```python
from build123d import *

# Parameters (mm, degrees)
F3_DEPTH     = 31.75
F5_DEPTH     = 6.35
F6_SIZE      = 12.7
F7_SIZE      = 12.7
F9_DEPTH     = 31.75
F11_DEPTH    = 12.7
F13_T2_ANGLE = 48.1784563201
F13_T4_ANGLE = 86.2150976381
F13_T6_ANGLE = 86.2150976381
F13_T8_ANGLE = 48.1784563201
F15_DEPTH    = 12.7
F16_SIZE     = 5.08
F18_DEPTH    = 2.54
F20_DEPTH    = 2.54
F21_R        = 7.62
F22_DEPTH    = 38.1
F24_DEPTH    = 2.794
F26_DEPTH    = 2.54
F27_R        = 10.16
F27_R_2      = 9.525
F28_DEPTH    = 76.2


# Not quite as in the source:
# - a fillet or chamfer that OpenCascade refuses, or shapes differently, is made with other operations: its cross-section is extruded or revolved along the edge and cut away or added
# - a feature of the source that left no trace in its solid (it failed there, or was rolled back) is left out
# - a feature names something its author has since deleted; it is built from what else it names


with BuildPart() as f3:
    # F2 (on Front) → F3 (new body, symmetric)
    with BuildSketch(Plane.XZ):
        with BuildLine():
            Line((37.9477068782, 57.15), (37.9477068782, -69.85))
            ThreePointArc((37.9477068782, -69.85), (197.3095607255, -116.6415507663), (342.7477068782, -196.85))
            Line((342.7477068782, -196.85), (342.7477068782, -156.4439684153))
            Line((342.7477068782, -156.4439684153), (333.764821291, -146.2200134993))
            Line((333.764821291, -146.2200134993), (333.764821291, -76.4565169811))
            Line((333.764821291, -76.4565169811), (299.7545793033, -41.7148783095))
            ThreePointArc((299.7545793033, -41.7148783095), (173.42869903, 19.8395158234), (37.9477068782, 57.15))
        make_face()
    extrude(amount=F3_DEPTH, both=True)

    # F4 (on Front) → F5 (cut, symmetric)
    with BuildSketch(Plane.XZ):
        with BuildLine():
            Line((37.9477068782, -48.4879799187), (37.9477068782, -69.85))
            ThreePointArc((37.9477068782, -69.85), (197.3095607255, -116.6415507663), (342.7477068782, -196.85))
            Line((342.7477068782, -196.85), (342.7477068782, -156.4439684153))
            Line((342.7477068782, -156.4439684153), (333.764821291, -146.2200134993))
            Line((333.764821291, -146.2200134993), (333.764821291, -76.4565169811))
            Line((333.764821291, -76.4565169811), (299.7545793033, -41.7148783095))
            ThreePointArc((299.7545793033, -41.7148783095), (173.42869903, 19.8395158234), (37.9477068782, 57.15))
            Line((37.9477068782, 57.15), (37.9477068782, 40.4159426689))
            ThreePointArc((37.9477068782, 40.4159426689), (174.1077804995, -9.1728518585), (291.3761138916, -94.3007096648))
            Line((291.3761138916, -94.3007096648), (297.9114055634, -145.1900005341))
            ThreePointArc((297.9114055634, -145.1900005341), (173.776538026, -81.1205697987), (37.9477068782, -48.4879799187))
        make_face()
    extrude(amount=F5_DEPTH, both=True, mode=Mode.SUBTRACT)

    # F6
    f6_edges = [f3.edges().sort_by_distance(p)[0] for p in [
        (173.428699, -31.75, 19.839516),
        (316.7597, -31.75, -59.085698),
        (316.7597, 31.75, -59.085698),
        (173.428699, 31.75, 19.839516),
    ]]
    chamfer(f6_edges, length=F6_SIZE)

    # F7
    f7_edges = [f3.edges().sort_by_distance(p)[0] for p in [
        (197.309561, -31.75, -116.641551),
        (197.309561, 31.75, -116.641551),
    ]]
    chamfer(f7_edges, length=F7_SIZE)

    # F8 (on Front) → F9 (join, symmetric)
    with BuildSketch(Plane.XZ):
        with BuildLine():
            ThreePointArc((86.9189181185, -80.2493599938), (62.5187399917, -74.647396796), (37.9477068782, -69.85))
            Line((37.9477068782, -69.85), (37.9477068782, -171.45))
            ThreePointArc((37.9477068782, -171.45), (117.3693749826, -201.1045334968), (188.127681613, -247.7998733521))
            ThreePointArc((188.127681613, -247.7998733521), (259.6802456544, -259.033648506), (329.51571574, -278.2423507795))
            Line((329.51571574, -278.2423507795), (342.7477068782, -203.2))
            ThreePointArc((342.7477068782, -203.2), (210.1366349445, -151.4972629597), (86.9189181185, -80.2493599938))
        make_face()
        with BuildLine():
            add(Edge.make_bspline(
                [(37.9477068782, -69.85), (37.9477068782, -67.7549506267), (37.9477068782, -65.6599012534), (37.9477068782, -63.5648518801)],
                knots=[0, 0, 0, 0, 0.4873412151, 0.4873412151, 0.4873412151, 0.4873412151], degree=3))
            ThreePointArc((37.9477068782, -69.85), (62.5187399917, -74.647396796), (86.9189181185, -80.2493599938))
            ThreePointArc((86.9189181185, -80.2493599938), (75.0688400161, -71.9981901024), (63.3477068782, -63.5648518801))
            Line((63.3477068782, -63.5648518801), (37.9477068782, -63.5648518801))
        make_face()
    extrude(amount=F9_DEPTH, both=True)

    # F10 (on Front) → F11 (cut, symmetric)
    with BuildSketch(Plane.XZ):
        with BuildLine():
            add(Edge.make_bspline(
                [(37.9477068782, -69.85), (37.9477068782, -67.7549506267), (37.9477068782, -65.6599012534), (37.9477068782, -63.5648518801)],
                knots=[0, 0, 0, 0, 0.4873412151, 0.4873412151, 0.4873412151, 0.4873412151], degree=3))
            Line((37.9477068782, -69.85), (37.9477068782, -171.45))
            ThreePointArc((37.9477068782, -171.45), (117.3693749826, -201.1045334968), (188.127681613, -247.7998733521))
            ThreePointArc((188.127681613, -247.7998733521), (259.6802456544, -259.033648506), (329.51571574, -278.2423507795))
            Line((329.51571574, -278.2423507795), (342.7477068782, -203.2))
            ThreePointArc((342.7477068782, -203.2), (197.1706361591, -145.1420264492), (63.3477068782, -63.5648518801))
            Line((63.3477068782, -63.5648518801), (37.9477068782, -63.5648518801))
        make_face()
    extrude(amount=F11_DEPTH, both=True, mode=Mode.SUBTRACT)

    # F13: chamfer of 76.2 x 19.05 on 4 edges, made by hand

    # F13_s1 → F13_t2 (revolve, cut)
    with BuildSketch(Plane(origin=(-60.6535291513, 0, -12.8240400006), x_dir=(0, 1, 0), z_dir=(-0.9783709739, 0, -0.2068580127))):
        Polygon((31.75, 174.9435450059), (12.7, 251.1435450059), (31.75, 251.1435450059), align=None)
    revolve(axis=Axis((124.3217755456, 31.75, -887.6969377111), (0, 1, 0)), revolution_arc=F13_T2_ANGLE, mode=Mode.SUBTRACT)

    # F13_s3 → F13_t4 (revolve, cut)
    with BuildSketch(Plane(origin=(-192.2531449662, 0, -55.7064857223), x_dir=(0, 1, 0), z_dir=(-0.9604918286, 0, -0.2783081876))):
        Polygon((12.7, 124.3402407106), (31.75, 48.1402407106), (31.75, 124.3402407106), align=None)
    revolve(axis=Axis((-53.0135938756, 31.75, -536.2473285656), (0, 1, 0)), revolution_arc=F13_T4_ANGLE, mode=Mode.SUBTRACT)

    # F13_s5 → F13_t6 (revolve, cut)
    with BuildSketch(Plane(origin=(-192.2531449662, 0, -55.7064857223), x_dir=(0, 1, 0), z_dir=(-0.9604918286, 0, -0.2783081876))):
        Polygon((-31.75, 48.1402407106), (-12.7, 124.3402407106), (-31.75, 124.3402407106), align=None)
    revolve(axis=Axis((-53.0135938756, -31.75, -536.2473285656), (0, 1, 0)), revolution_arc=F13_T6_ANGLE, mode=Mode.SUBTRACT)

    # F13_s7 → F13_t8 (revolve, cut)
    with BuildSketch(Plane(origin=(-60.6535291513, 0, -12.8240400006), x_dir=(0, 1, 0), z_dir=(-0.9783709739, 0, -0.2068580127))):
        Polygon((-31.75, 174.9435450059), (-12.7, 251.1435450059), (-31.75, 251.1435450059), align=None)
    revolve(axis=Axis((124.3217755456, -31.75, -887.6969377111), (0, 1, 0)), revolution_arc=F13_T8_ANGLE, mode=Mode.SUBTRACT)

    # F14 (on Front) → F15 (join, symmetric)
    with BuildSketch(Plane.XZ):
        with BuildLine():
            Line((354.91571574, -208.3923507795), (354.91571574, -113.1423507795))
            ThreePointArc((354.91571574, -113.1423507795), (259.66571574, -208.3923507795), (354.91571574, -303.6423507795))
            Line((354.91571574, -303.6423507795), (354.91571574, -208.3923507795))
        make_face()
    extrude(amount=F15_DEPTH, both=True)

    # F16
    f16_edges = [f3.edges().sort_by_distance(p)[0] for p in [
        (310.909323, -12.7, -292.867199),
        (270.087911, -12.7, -165.070232),
        (344.273637, -12.7, -113.738726),
        (344.273637, 12.7, -113.738726),
        (270.087911, 12.7, -165.070232),
        (310.909323, 12.7, -292.867199),
    ]]
    chamfer(f16_edges, length=F16_SIZE)

    # F17 (on face) → F18 (cut)
    with BuildSketch(Plane.XZ.offset(31.75)):
        with BuildLine():
            Line((37.9477068782, 18.4170784308), (37.9477068782, -18.7770907031))
            Line((37.9477068782, -18.7770907031), (44.5238578239, -19.4250085564))
            ThreePointArc((44.5238578239, -19.4250085564), (166.0160786587, -50.5371993601), (281.275870441, -99.9690568843))
            Line((281.275870441, -99.9690568843), (270.4956403873, -68.620350335))
            ThreePointArc((270.4956403873, -68.620350335), (157.9813255542, -15.0565404403), (37.9477068782, 18.4170784308))
        make_face()
    extrude(amount=-F18_DEPTH, mode=Mode.SUBTRACT)

    # F19 (on face) → F20 (cut)
    with BuildSketch(Plane(origin=(0, 31.75, 0), x_dir=(-1, 0, 0), z_dir=(0, 1, 0))):
        with BuildLine():
            ThreePointArc((-37.9477068782, 18.4170784308), (-157.9813255542, -15.0565404403), (-270.4956403873, -68.620350335))
            Line((-270.4956403873, -68.620350335), (-281.275870441, -99.9690568843))
            ThreePointArc((-281.275870441, -99.9690568843), (-166.0160786587, -50.5371993601), (-44.5238578239, -19.4250085564))
            Line((-44.5238578239, -19.4250085564), (-37.9477068782, -18.7770907031))
            Line((-37.9477068782, -18.7770907031), (-37.9477068782, 18.4170784308))
        make_face()
    extrude(amount=-F20_DEPTH, mode=Mode.SUBTRACT)

    # F21 (on face) → F22 (cut)
    with BuildSketch(Plane.YZ.offset(354.91571574)):
        with Locations((0, -208.3923507795)):
            Circle(F21_R)
    extrude(amount=-F22_DEPTH, mode=Mode.SUBTRACT)

    # F23 (on face) → F24 (cut)
    with BuildSketch(Plane.XZ.offset(12.7)):
        with BuildLine():
            ThreePointArc((331.4293971954, -267.3893239326), (342.9586633277, -270.7564341738), (354.91571574, -271.8923507795))
            Line((354.91571574, -271.8923507795), (354.91571574, -259.1923507795))
            ThreePointArc((354.91571574, -259.1923507795), (344.0535486893, -258.0174787588), (333.6938090461, -254.5472061718))
            Line((333.6938090461, -254.5472061718), (331.4293971954, -267.3893239326))
        make_face()
        with BuildLine():
            ThreePointArc((342.7477068782, -159.0711630369), (348.7869449547, -157.9634090034), (354.91571574, -157.5923507795))
            Line((354.91571574, -157.5923507795), (354.91571574, -144.8923507795))
            ThreePointArc((354.91571574, -144.8923507795), (344.9966028413, -145.6718501493), (335.3210156829, -147.991210644))
            Line((335.3210156829, -147.991210644), (342.7477068782, -156.4439684153))
            Line((342.7477068782, -156.4439684153), (342.7477068782, -159.0711630369))
        make_face()
        with BuildLine():
            ThreePointArc((303.5618689691, -171.0422179573), (298.710555552, -178.8418860075), (295.0352686554, -187.2598625929))
            ThreePointArc((295.0352686554, -187.2598625929), (301.0091143651, -189.413157651), (306.9974582895, -191.5257979926))
            ThreePointArc((306.9974582895, -191.5257979926), (310.1473048853, -184.3834068306), (314.3542442481, -177.8079261419))
            ThreePointArc((314.3542442481, -177.8079261419), (308.9721939736, -174.4025207151), (303.5618689691, -171.0422179573))
        make_face()
    extrude(amount=-F24_DEPTH, mode=Mode.SUBTRACT)

    # F25 (on face) → F26 (cut)
    with BuildSketch(Plane(origin=(0, 12.7, 0), x_dir=(-1, 0, 0), z_dir=(0, 1, 0))):
        with BuildLine():
            Line((-354.91571574, -259.1923507795), (-354.91571574, -271.8923507795))
            ThreePointArc((-354.91571574, -271.8923507795), (-342.9586633277, -270.7564341738), (-331.4293971954, -267.3893239326))
            Line((-331.4293971954, -267.3893239326), (-333.6938090461, -254.5472061718))
            ThreePointArc((-333.6938090461, -254.5472061718), (-344.0535486893, -258.0174787588), (-354.91571574, -259.1923507795))
        make_face()
        with BuildLine():
            ThreePointArc((-335.3210156829, -147.991210644), (-344.9966028413, -145.6718501493), (-354.91571574, -144.8923507795))
            Line((-354.91571574, -144.8923507795), (-354.91571574, -157.5923507795))
            ThreePointArc((-354.91571574, -157.5923507795), (-348.7869449547, -157.9634090034), (-342.7477068782, -159.0711630369))
            Line((-342.7477068782, -159.0711630369), (-342.7477068782, -156.4439684153))
            Line((-342.7477068782, -156.4439684153), (-335.3210156829, -147.991210644))
        make_face()
        with BuildLine():
            ThreePointArc((-295.0352686554, -187.2598625929), (-298.710555552, -178.8418860075), (-303.5618689691, -171.0422179573))
            ThreePointArc((-303.5618689691, -171.0422179573), (-308.9721939736, -174.4025207151), (-314.3542442481, -177.8079261419))
            ThreePointArc((-314.3542442481, -177.8079261419), (-310.1473048853, -184.3834068306), (-306.9974582895, -191.5257979926))
            ThreePointArc((-306.9974582895, -191.5257979926), (-301.0091143651, -189.413157651), (-295.0352686554, -187.2598625929))
        make_face()
    extrude(amount=-F26_DEPTH, mode=Mode.SUBTRACT)

    # F27 (on face) → F28 (cut)
    with BuildSketch(Plane(origin=(0, 0, 0), x_dir=(0, -1, 0), z_dir=(-1, 0, 0))):
        Circle(F27_R)
        Circle(F27_R_2, mode=Mode.SUBTRACT)
        Circle(F27_R_2)
    extrude(amount=-F28_DEPTH, mode=Mode.SUBTRACT)


solid = f3.part
```
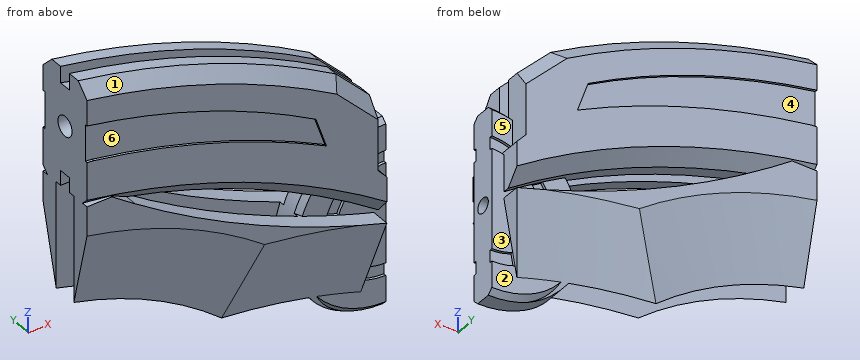
The listing builds one solid part. Answer for the finished solid, in the listing's coordinates (mm). Face numbers are marked on the shaded views. A direction names the side the tool comes from. Round coordinates to 2 decimals unless told otherwise and drop trailing zeros. Loops run counter-clockwise (first coordinate to the right, second up) from the corner with the lowest first, then second, coordinate; pieces in that order, holes last.
1) For a pull along Z with two mould halves and no side action, classify the marked faces 1, 2 and 3 as released by +Z, released by -Z, zero draft, split by the parting line, or undercut.
Outcome:
face 1: released by +Z
face 2: zero draft
face 3: undercut
2) Given P1, Ø1.9, axis at x = 51, y = -10.5, coming from the -Z side; P2, Ø14.5, axis at x = 339.5, z = -200, coming from the -Y side; P3, Ø19, axis at x = 337.5, z = -265, coming from the +Y side, each flat-ended and moving along its own axis, determine where each tip first touches the part or whether it passes through.
Outcome:
P1: stops at z = -63.56
P2: stops at y = -31.56
P3: stops at y = 18.17
3) For the marked faces 4, 5 and 6, determine the directions among +Z, -Z, +X, -X, +Y, -Y from which every point of the face is accessible in a straight line to the end or side of a thin tool.
Outcome:
face 4: +Y
face 5: +Z, +X, +Y
face 6: -Y
4) A cutting plane is placed at A-A on y = 0. Determine the outline of the cut face in (x, z).
Outcome:
outline: (37.95, -48.49) arc R581.8 cw to (289.24, -139.41) arc R95.25 ccw to (354.92, -303.64) - (354.92, -216.01) - (316.82, -216.01) - (316.82, -200.77) - (354.92, -200.77) - (354.92, -113.14) arc R95.25 ccw to (296.38, -133.25) - (291.38, -94.3) arc R521.73 ccw to (37.95, 40.42) - (37.95, 10.16) - (76.2, 10.16) - (76.2, -10.16) - (37.95, -10.16) - close
5) Consider line 1 (X direction, y = 11.5, z = -37); line 2 (Z direction, x = 67.5, y = 0); line 3 (Z direction, x = 269.5, y = 12.5). Determine where each line is inside the solid, lowest interval first.
Outcome:
line 1: x = 37.95 to 291.88
line 2: z = -52.69 to -10.16, 10.16 to 33.21
line 3: z = -250.54 to -177.53, -151.28 to -24.28
